Read the model definition and answer for the solid it produces. Units are mm, in the model's axes. Face numbers are marked on the shaded views. Give positions to 0.01 mm unless a question says otherwise; leave off trailing zeros. Write each loop counter-clockwise with the first axis right and the second up, starting at its lowest first coordinate (ties: lowest second). Pieces come first, ordered by that corner, then holes. Notation, with made-up numbers: (-31, -38) -> (24, -38) arc R27 ccw to (24, -9) -> close; hole circle Ø10 at (0.25, 7.5). An arc over 180 degrees is marked (long way). Answer as CSV lines item,"result". Start each with the question number.
1. The part is cut by section B-B, the plane y = -20. Determine the outline of the cut face in (x, z), and give its area (3 significant figures).
2. The part is cut by section C-C, the plane x = -1.5. Determine the outline of the cut face in (y, z), and give its area (3 significant figures).
3. For a pull along X with two mould halves and no side action, classify the marked faces 1, 2 and 3 as pulls with the +X half, pulls with the -X half, needs draft (parallel to the pull), parting line crosses it, or undercut.
4. Given pin 1 (8 mm diameter, centred on x = -12, y = -72.5, fed in from +Z); pin 2 (4 mm diameter, centred on x = -2, y = -71.5, fed in from -Z); pin 3 (2 mm diameter, centred on x = 6, y = -49.5, fed in from +Z), each flat-ended and moving along its own axis, determine where each tip first touches the part or whether it passes through.
5. Find the intervals of material crossed by line 1 (X direction, y = -8, z = -8.25); line 2 (X direction, y = -65.5, z = -4.5); line 3 (Z direction, x = -2.5, y = -86), in increasing order.
6. The part is cut by section A-A, the plane z = -7.5. Determine the outline of the cut face in (x, y), and give its area (3 significant figures).
from build123d import *

# Parameters (mm, degrees)
F1_DEPTH = 102.87


with BuildPart() as f1:
    # F0 (on Front) → F1 (new body)
    with BuildSketch(Plane.XZ):
        with BuildLine():
            Line((22.606, -13.555481), (3.550875, -0.702637))
            ThreePointArc((3.550875, -0.702637), (1.85656, 0.105509), (0, 0.382974))
            ThreePointArc((0, 0.382974), (-1.85656, 0.105509), (-3.550875, -0.702637))
            Line((-3.550875, -0.702637), (-22.606, -13.555481))
            Line((-22.606, -13.555481), (-22.606, -13.938456))
            Line((-22.606, -13.938456), (-3.550875, -1.085611))
            ThreePointArc((-3.550875, -1.085611), (-1.85656, -0.277465), (0, 0))
            ThreePointArc((0, 0), (1.85656, -0.277465), (3.550875, -1.085611))
            Line((3.550875, -1.085611), (22.606, -13.938456))
            Line((22.606, -13.938456), (22.606, -13.555481))
        make_face()
    extrude(amount=F1_DEPTH)


solid = f1.part
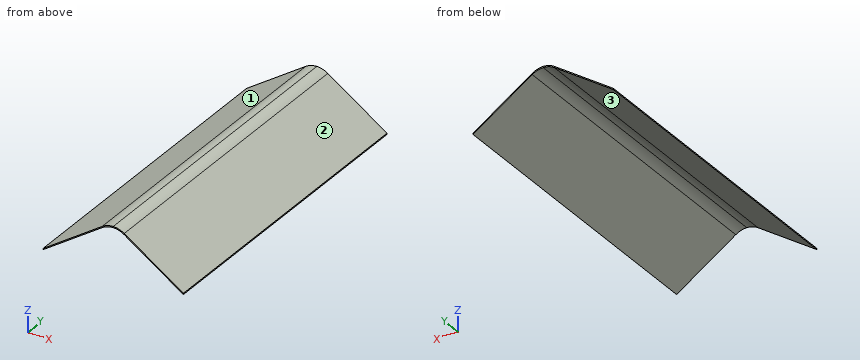
Results found:
1,outline,"(-22.61, -13.94) -> (-3.55, -1.09) arc R6.35 cw to (0, 0) arc R6.35 cw to (3.55, -1.09) -> (22.61, -13.94) -> (22.61, -13.56) -> (3.55, -0.7) arc R6.35 ccw to (0, 0.38) arc R6.35 ccw to (-3.55, -0.7) -> (-22.61, -13.56) -> close"
1,area,"17.3 mm²"
2,outline,"(-102.87, -0.18) -> (0, -0.18) -> (0, 0.2) -> (-102.87, 0.2) -> close"
2,area,"39.4 mm²"
3,face 1,"pulls with the -X half"
3,face 2,"pulls with the +X half"
3,face 3,"undercut"
4,pin 1,"stops at z = -3.7"
4,pin 2,"stops at z = -1.39"
4,pin 3,"stops at z = -1.68"
5,line 1,"x = -14.74 to -14.17, 14.17 to 14.74"
5,line 2,"x = -9.18 to -8.61, 8.61 to 9.18"
5,line 3,"z = -0.51 to -0.13"
6,outline,"(-13.63, -102.87) -> (-13.06, -102.87) -> (-13.06, 0) -> (-13.63, 0) -> close; (13.06, -102.87) -> (13.63, -102.87) -> (13.63, 0) -> (13.06, 0) -> close"
6,area,"117 mm²"
